Autodesk Inventor part; units mm, degrees
ref_plane "YZ Plane" through (0, 0, 0) normal (1, 0, 0) x (0, 1, 0)
ref_plane "XZ Plane" through (0, 0, 0) normal (0, 1, 0) x (-1, 0, 0)
ref_plane "XY Plane" through (0, 0, 0) normal (0, 0, 1) x (1, 0, 0)
sketch "Sketch1" plane through (0, 0, 0) normal (0, 0, 1) x (1, 0, 0)
  circle A0 centre (0, 0) radius 5.15
  dimension "d0" = 10.3
extrude "Extrusion1" add sketch "Sketch1" along normal blind 2.3
sketch "Sketch2" plane through (0, 0, 2.3) normal (0, 0, 1) x (1, 0, 0)
  circle A0 centre (0, 0) radius 6.2
  dimension "d3" = 12.4
extrude "Extrusion2" add sketch "Sketch2" along normal blind 1
sketch "Sketch3" plane through (0, 0, 2.3) normal (0, 0, -1) x (-1, 0, 0)
  circle A0 centre (0, 0) radius 6.2 construction
  line L0 (6.2, 0) -> (3.7, 0)
  line L1 (3.7, 0) -> (3.7, 5.5)
  line L2 (3.7, 5.5) -> (6.2, 5.5)
  line L3 (6.2, 5.5) -> (6.2, 0)
  line L4 (0, -6.2) -> (0, 6.2)
  circle A1 centre (0, 0) radius 6.2 construction
  line L5 (-6.2, 0) -> (-3.7, 0)
  line L6 (-3.7, 0) -> (-3.7, 5.5)
  line L7 (-3.7, 5.5) -> (-6.2, 5.5)
  line L8 (-6.2, 5.5) -> (-6.2, 0)
  dimension "d6" = 5.5
  dimension "d7" = 2.5
extrude "Extrusion3" add sketch "Sketch3" against normal blind 5.5
sketch "Sketch4" plane through (6.2, 0, 2.3) normal (1, 0, 0) x (0, 0, -1)
  line L0 (0, 5.5) -> (0, 0) construction
  line L1 (0, 5.5) -> (-5.5, 5.5) construction
  line L2 (-5.5, 0) -> (-5.5, 5.5) construction
  line L3 (-1, 0) -> (-5.5, 0) construction
  line L4 (0, 0) -> (-1, 0) construction
  line L5 (-5.5, 0) -> (-5.5, 5.5) construction
  line L6 (0, 5.5) -> (-5.5, 0) construction
  line L7 (0, -6.2) -> (0, 0) construction
  line L8 (-5.5, 5.5) -> (0, 0) construction
  circle A0 centre (-2.75, 2.75) radius 1.6
  point P0 (2.3, 0)
  dimension "d10" = 3.2
extrude "Extrusion4" cut sketch "Sketch4" against normal through all
fillet "Fillet1" radius 1 2 edges at (4.95, 0, 7.8) (-4.95, 0, 7.8)
sketch "Sketch5" plane through (0, 0, 7.8) normal (0, 0, 1) x (1, 0, 0)
  line L0 (6.2, 1) -> (3.7, 1) construction
  line L1 (6.2, 1) -> (6.2, 5.5) construction
  line L2 (6.2, 5.5) -> (3.7, 5.5) construction
  line L3 (3.7, 5.5) -> (3.7, 1) construction
  line L4 (-3.7, 1) -> (-6.2, 1) construction
  line L5 (-3.7, 1) -> (-3.7, 5.5) construction
  line L6 (-3.7, 5.5) -> (-6.2, 5.5) construction
  line L7 (-6.2, 5.5) -> (-6.2, 1) construction
  line L8 (6.2, 5.5) -> (6.2, 0)
  line L9 (-6.2, 5.5) -> (-6.2, 0)
  line L10 (6.2, 5.5) -> (-6.2, 5.5)
  line L11 (-6.2, 5.5) -> (-6.2, 2.5)
  line L12 (-6.2, 2.5) -> (6.2, 2.5)
  line L13 (6.2, 2.5) -> (6.2, 5.5)
  point P0 (0, 0)
  dimension "d14" = 3
extrude "Extrusion5" add sketch "Sketch5" along normal blind 8
fillet "Fillet2" radius 1 2 edges at (-4.95, 2.5, 7.8) (4.95, 2.5, 7.8)
fillet "Fillet3" radius 4 2 edges at (-6.2, 4, 15.8) (6.2, 4, 15.8)
sketch "Sketch6" plane through (-3.7, 2.5, 7.8) normal (0, -1, 0) x (1, 0, 0)
  line L0 (3.7, -7.8) -> (3.7, 7.2594)
  line L1 (0, 0) -> (7.4, 0) construction
  arc A0 (9.9, 4) -> (5.9, 8) centre (5.9, 4) ccw construction
  line L2 (1.5, 8) -> (5.9, 8) construction
  arc A1 (1.5, 8) -> (-2.5, 4) centre (1.5, 4) ccw construction
  line L3 (-2.5, 1) -> (-2.5, 4) construction
  line L4 (0, 1) -> (-2.5, 1) construction
  line L5 (0, 1) -> (0, 0) construction
  line L6 (0, 0) -> (7.4, 0) construction
  line L7 (7.4, 0) -> (7.4, 1) construction
  line L8 (9.9, 1) -> (7.4, 1) construction
  line L9 (9.9, 1) -> (9.9, 4) construction
  line L10 (-6.2522, 4) -> (14.3588, 4) construction
  circle A2 centre (3.7, 4) radius 1.6
  circle A3 centre (3.7, 4) radius 4 construction
  dimension "d19" = 4
  dimension "d20" = 3.2
  dimension "d23" = 8
extrude "Extrusion6" cut sketch "Sketch6" against normal through all
properties part number "magnet-holder-end"
Work out the finished part from the listing and answer in its coordinate system (mm). A direction names the side the tool comes from. Give positions to 0.01 mm unless a question says otherwise; leave off trailing zeros. Write each loop counter-clockwise with the first axis right and the second up, starting at its lowest first coordinate (ties: lowest second). Pieces come first, ordered by that corner, then holes.
(1) Which of the six approach directions +Z, -Z, +X, -X, +Y, -Y give full straight-line access (tool end or side, diameter ignored) to faces 1 (the flat face through (0, 4, 7.8)), 2 (the flat face through (0, 0, 3.3)), 3 (the flat face through (-5, 0, 5)), 4 (the cylindrical face through (4.91, -1.55, 1.13))?
Final values:
face 1: +Y, -Y
face 2: -Y
face 3: +Z, +X, -X, -Y
face 4: -Z
(2) Straight lines are drawn through the part: line 1 (Y direction, x = 4.6, z = 5.05); line 2 (Z direction, x = 0, y = 3.4); line 3 (X direction, y = 4, z = 6.25). For each, find the intervals that lie inside material, in ascending order.
Final values:
line 1: y = 0 to 1.15, 4.35 to 5.5
line 2: z = 0 to 3.3, 7.8 to 10.2, 13.4 to 15.8
line 3: x = -6.2 to -3.7, 3.7 to 6.2
(3) Flat-ended cylindrical pins translate along their axes: pin 1 Ø0.6 at (x, y) = (5, 1.5) entering from +Z; pin 2 Ø2 at (x, z) = (5, 5) entering from -Y; pin 3 Ø4 at (y, z) = (2.75, 5.05) entering from -X; pin 4 Ø6.5 at (x, z) = (1, 13.5) entering from -Y. Find the tip coordinate at first contact, or state that the pin passes through.
Final values:
pin 1: stops at z = 7.85
pin 2: stops at y = 0
pin 3: stops at x = -6.2
pin 4: stops at y = 2.5
(4) The mould has two halves that part along Z. Classify faces 5 (the flat face through (0, 5.5, 9)), 6 (the cylindrical face through (-0.208, 3.979, 13.386)), 7 (the cylindrical face through (4.968, 2.199, 8.085)): pulls with the +Z half, pulls with the -Z half, needs draft (parallel to the pull), parting line crosses it, or undercut.
Final values:
face 5: needs draft
face 6: undercut
face 7: pulls with the +Z half
(5) The part is cut by section B-B on z = 5.05. Write down the section's boundary in (x, y), plus the area to 3 significant figures.
Final values:
outline: (-6.2, 0) - (-3.7, 0) - (-3.7, 1.15) - (-6.2, 1.15) - close; (-6.2, 4.35) - (-3.7, 4.35) - (-3.7, 5.5) - (-6.2, 5.5) - close; (3.7, 0) - (6.2, 0) - (6.2, 1.15) - (3.7, 1.15) - close; (3.7, 4.35) - (6.2, 4.35) - (6.2, 5.5) - (3.7, 5.5) - close
area: 11.5 mm2
(6) The part is cut by section C-C on y = 3. Write down the section's boundary in (x, z), plus the area to 3 significant figures.
Final values:
outline: (-6.2, 2.3) - (-4.19, 2.3) - (-4.19, 0) - (4.19, 0) - (4.19, 2.3) - (6.2, 2.3) - (6.2, 3.47) - (3.7, 3.47) - (3.7, 3.3) - (-3.7, 3.3) - (-3.7, 3.47) - (-6.2, 3.47) - close; (-6.2, 6.63) - (-3.7, 6.63) - (-3.7, 7.8) - (3.7, 7.8) - (3.7, 6.63) - (6.2, 6.63) - (6.2, 11.8) arc R4 ccw to (2.2, 15.8) - (-2.2, 15.8) arc R4 ccw to (-6.2, 11.8) - close; hole circle Ø3.2 at (0, 11.8)
area: 123 mm2
(7) The part is cut by section A-A on x = 0. Write down the section's boundary in (y, z), plus the area to 3 significant figures.
Final values:
outline: (-6.2, 2.3) - (-5.15, 2.3) - (-5.15, 0) - (5.15, 0) - (5.15, 2.3) - (6.2, 2.3) - (6.2, 3.3) - (-6.2, 3.3) - close; (2.5, 7.8) - (5.5, 7.8) - (5.5, 10.2) - (2.5, 10.2) - close; (2.5, 13.4) - (5.5, 13.4) - (5.5, 15.8) - (2.5, 15.8) - close
area: 50.5 mm2
(8) The part is cut by section D-D on y = 1.75. Write down the section's boundary in (x, z).
Final values:
outline: (-6.2, 2.3) - (-4.84, 2.3) - (-4.84, 0) - (4.84, 0) - (4.84, 2.3) - (6.2, 2.3) - (6.2, 3.8) - (3.7, 3.8) - (3.7, 3.3) - (-3.7, 3.3) - (-3.7, 3.8) - (-6.2, 3.8) - close; (-6.2, 6.3) - (-3.7, 6.3) - (-3.7, 7.83) - (-6.2, 7.83) - close; (3.7, 6.3) - (6.2, 6.3) - (6.2, 7.83) - (3.7, 7.83) - close
